from build123d import *

# Parameters (mm, degrees)
SKETCH1_W                 = 30
SKETCH1_H                 = 35
BOSS_EXTRUDE1_DEPTH       = 8
SKETCH3_W                 = 29
SKETCH3_H                 = 5
CUT_EXTRUDE1_DEPTH        = 68
SKETCH4_W                 = 20
SKETCH4_H                 = 2
BOSS_EXTRUDE2_DEPTH       = 6
SKETCH5_W                 = 20
SKETCH5_H                 = 2
BOSS_EXTRUDE3_DEPTH       = 6
F_3_0MM_DOWEL_HOLE1_D     = 3
F_3_0MM_DOWEL_HOLE1_DEPTH = 12
F_3_0MM_DOWEL_HOLE1_TIP   = 0.901290929


with BuildPart() as part:
    # Sketch1 → Boss-Extrude1 (new body)
    with BuildSketch(Plane(origin=(0, 0, 0), x_dir=(1, 0, 0), z_dir=(0, 1, 0))):
        with Locations((-15, 17.5)):
            Rectangle(SKETCH1_W, SKETCH1_H)
    extrude(amount=BOSS_EXTRUDE1_DEPTH)

    # Sketch3 → Cut-Extrude1 (cut)
    with BuildSketch(Plane(origin=(0, 0, 0), x_dir=(0, 0, -1), z_dir=(1, 0, 0))):
        with Locations((17.5, 2.5)):
            Rectangle(SKETCH3_W, SKETCH3_H)
    extrude(amount=-CUT_EXTRUDE1_DEPTH, mode=Mode.SUBTRACT)

    # Sketch4 → Boss-Extrude2 (add)
    with BuildSketch(Plane.XY):
        with Locations((-15, 1)):
            Rectangle(SKETCH4_W, SKETCH4_H)
    extrude(amount=BOSS_EXTRUDE2_DEPTH)

    # Sketch5 → Boss-Extrude3 (add)
    with BuildSketch(Plane(origin=(0, 0, -35), x_dir=(-1, 0, 0), z_dir=(0, 0, -1))):
        with Locations((15, 1)):
            Rectangle(SKETCH5_W, SKETCH5_H)
    extrude(amount=BOSS_EXTRUDE3_DEPTH)

    # Ø3.0mm Dowel Hole1
    with Locations(Plane.XZ):
        with Locations((-15, -38), (-15, 3)):
            Hole(F_3_0MM_DOWEL_HOLE1_D / 2, depth=F_3_0MM_DOWEL_HOLE1_DEPTH)
            with Locations((0, 0, -(F_3_0MM_DOWEL_HOLE1_DEPTH + F_3_0MM_DOWEL_HOLE1_TIP / 2))):  # 118° drill point
                Cone(0, F_3_0MM_DOWEL_HOLE1_D / 2, F_3_0MM_DOWEL_HOLE1_TIP, mode=Mode.SUBTRACT)


solid = part.part
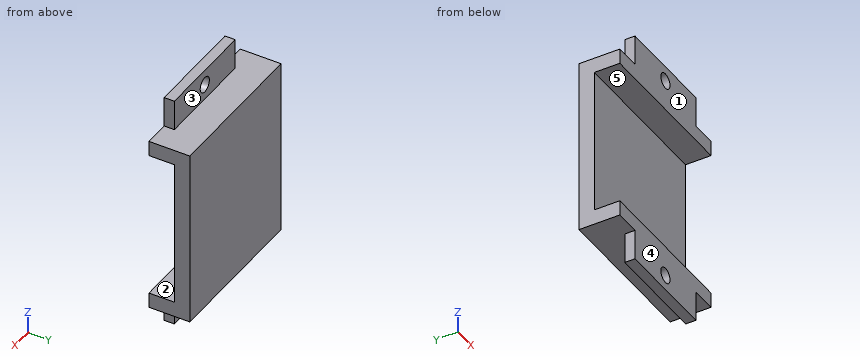
Verification items for the finished model (mm, model axes). Face numbers are marked on the shaded views. A direction names the side the tool comes from. Give positions to 0.01 mm unless a question says otherwise; leave off trailing zeros. Write each loop counter-clockwise with the first axis right and the second up, starting at its lowest first coordinate (ties: lowest second). Pieces come first, ordered by that corner, then holes.
(1) Gauge pin test, flat ends, axial feed: pin 1 (2.5 mm diameter, centred on x = -15, z = -38, fed in from +Y); pin 2 (5 mm diameter, centred on x = -17, z = -38.5, fed in from +Y); pin 3 (0.6 mm diameter, centred on y = 1, z = -37, fed in from +X); pin 4 (1 mm diameter, centred on x = -4, y = 5.5, fed in from +Z). Record the tip position at first contact, or that the pin passes through.
(2) Material ranges on line 1 (Z direction, x = -15, y = 0.4); line 2 (Z direction, x = -17.5, y = 1.25); line 3 (Z direction, x = -15.5, y = 2.5), recorded low to high.
(3) Cross-section at C-C (z = 3). Enter the section's corners in (x, y), plus the area to 3 significant figures.
(4) Mould release check, pull along Z, two halves, no side actions. Record for the marked faces 4 and 5: +Z half, -Z half, draft (parallel to the pull), parting line (faces both ways), or undercut.
(5) Access from +Z, -Z, +X, -X, +Y, -Y to the whole of each face (thin tool, end or side, straight path). Record for the marked faces 1, 2 and 3.
(6) Cross-section at A-A (y = 1.25). Enter the section's corners in (x, z), plus the area to 3 significant figures.
(7) Cross-section at D-D (x = -11). Enter the section's corners in (y, z).
(8) Cross-section at B-B (x = -15). Enter the section's corners in (y, z).
Worked out:
1. pin 1: passes through
1. pin 2: stops at y = 2
1. pin 3: stops at x = -5
1. pin 4: stops at z = 0
2. line 1: z = -41 to -39.5, -36.5 to -32, -3 to 1.5, 4.5 to 6
2. line 2: z = -41 to -32, -3 to 6
2. line 3: z = -35 to -32, -3 to 0
3. outline: (-25, 0) - (-16.5, 0) - (-16.5, 2) - (-25, 2) - close; (-13.5, 0) - (-5, 0) - (-5, 2) - (-13.5, 2) - close
3. area: 34.0 mm2
4. face 4: draft
4. face 5: undercut
5. face 1: +Z, -Z, +X, -X, -Y
5. face 2: +X, -X, -Y
5. face 3: +Z, +X, -X, +Y
6. outline: (-30, -35) - (-25, -35) - (-25, -41) - (-5, -41) - (-5, -35) - (0, -35) - (0, -32) - (-30, -32) - close; (-30, -3) - (0, -3) - (0, 0) - (-5, 0) - (-5, 6) - (-25, 6) - (-25, 0) - (-30, 0) - close; hole circle Ø3 at (-15, -38); hole circle Ø3 at (-15, 3)
6. area: 406 mm2
7. outline: (0, -41) - (2, -41) - (2, -35) - (8, -35) - (8, 0) - (2, 0) - (2, 6) - (0, 6) - (0, -3) - (5, -3) - (5, -32) - (0, -32) - close
8. outline: (0, -41) - (2, -41) - (2, -39.5) - (0, -39.5) - close; (0, -36.5) - (2, -36.5) - (2, -35) - (8, -35) - (8, 0) - (2, 0) - (2, 1.5) - (0, 1.5) - (0, -3) - (5, -3) - (5, -32) - (0, -32) - close; (0, 4.5) - (2, 4.5) - (2, 6) - (0, 6) - close
